Read the model definition and answer for the solid it produces. Units are mm, in the model's axes. A direction names the side the tool comes from. Coordinates: 2 decimals unless noted, no trailing zeros. Write each loop counter-clockwise with the first axis right and the second up, starting at its lowest first coordinate (ties: lowest second). Pieces come first, ordered by that corner, then holes. Notation, with made-up numbers: M 70.25,3.25 L 109.25,3.25 A20 ccw 109.25,26.25 Z; hole C -21,69 d4. An arc over 180 degrees is marked long. Write item = value, one per line.
from build123d import *

# Parameters (mm, degrees)
SKETCH1_W           = 61
SKETCH1_H           = 57
BOSS_EXTRUDE1_DEPTH = 2
FILLET1_R           = 2.5
SKETCH2_R           = 1.25
CUT_EXTRUDE1_DEPTH  = 2
SKETCH3_W           = 31
SKETCH3_H           = 1
CUT_EXTRUDE2_DEPTH  = 2


with BuildPart() as part:
    # Sketch1 → Boss-Extrude1 (new body)
    with BuildSketch(Plane.XY):
        Rectangle(SKETCH1_W, SKETCH1_H)
    extrude(amount=BOSS_EXTRUDE1_DEPTH)

    # Fillet1
    fillet1_edges = [part.edges().sort_by_distance(p)[0] for p in [
        (30.5, -28.5, 1),
        (-30.5, -28.5, 1),
        (-30.5, 28.5, 1),
        (30.5, 28.5, 1),
    ]]
    fillet(fillet1_edges, radius=FILLET1_R)

    # Sketch2 → Cut-Extrude1 (cut)
    with BuildSketch(Plane.XY.offset(2)):
        with Locations((-26.25, 24.5)):
            Circle(SKETCH2_R)
        with Locations((-8.75, 24.5)):
            Circle(SKETCH2_R)
        with Locations((8.75, 24.5)):
            Circle(SKETCH2_R)
        with Locations((26.25, 24.5)):
            Circle(SKETCH2_R)
        with Locations((26.25, 8.166666667)):
            Circle(SKETCH2_R)
        with Locations((26.25, -8.166666667)):
            Circle(SKETCH2_R)
        with Locations((-8.75, -24.5)):
            Circle(SKETCH2_R)
        with Locations((8.75, -24.5)):
            Circle(SKETCH2_R)
        with Locations((26.25, -24.5)):
            Circle(SKETCH2_R)
        with Locations((-26.25, 8.166666667)):
            Circle(SKETCH2_R)
        with Locations((-26.25, -8.166666667)):
            Circle(SKETCH2_R)
        with Locations((-26.25, -24.5)):
            Circle(SKETCH2_R)
    extrude(amount=-CUT_EXTRUDE1_DEPTH, mode=Mode.SUBTRACT)

    # Sketch3 → Cut-Extrude2 (cut)
    with BuildSketch(Plane.XY.offset(2)):
        Rectangle(SKETCH3_W, SKETCH3_H)
        with Locations((0, -2.5)):
            Rectangle(SKETCH3_W, SKETCH3_H)
        with Locations((0, -5)):
            Rectangle(SKETCH3_W, SKETCH3_H)
        with Locations((0, -7.5)):
            Rectangle(SKETCH3_W, SKETCH3_H)
        with Locations((0, -10)):
            Rectangle(SKETCH3_W, SKETCH3_H)
    extrude(amount=-CUT_EXTRUDE2_DEPTH, mode=Mode.SUBTRACT)


solid = part.part
Item 1: Find section C-C (x = 26.25). Determine the outline of the cut face in (y, z).
Worked answers:
outline = M -28.5,0 L -25.75,0 L -25.75,2 L -28.5,2 Z; M -23.25,0 L -9.42,0 L -9.42,2 L -23.25,2 Z; M -6.92,0 L 6.92,0 L 6.92,2 L -6.92,2 Z; M 9.42,0 L 23.25,0 L 23.25,2 L 9.42,2 Z; M 25.75,0 L 28.5,0 L 28.5,2 L 25.75,2 Z
Item 2: Find section A-A (x = -8.75). State how many separate pieces and enclosed holes the cut face has, and give its area (3 significant figures).
Worked answers:
separate_pieces = 8
enclosed_holes = 0
area = 94.0 mm²
Item 3: For a pull along Y with two mould halves and no side action, classify faces 3 (the face through (30.5, 0, 1)), 4 (the face through (7.76, -25.26, 1.01)), 5 (the face through (-29.787, 27.748, 1.014)) as released by +Y, released by -Y, zero draft, split by the parting line, or undercut.
Worked answers:
face_3 = zero draft
face_4 = undercut
face_5 = released by +Y
Item 4: Consider line 1 along Y through (x, z) = (11, 0.85); line 2 along Y through (x, z) = (26.25, 0.7); line 3 along X through (y, z) = (-25.5, 1.8). Determine where each line is inside the solid, lowest interval first. Write a range as from..to.
Worked answers:
line_1 = -28.5..-10.5, -9.5..-8, -7..-5.5, -4.5..-3, -2..-0.5, 0.5..28.5
line_2 = -28.5..-25.75, -23.25..-9.42, -6.92..6.92, 9.42..23.25, 25.75..28.5
line_3 = -30.5..-27, -25.5..-9.5, -8..8, 9.5..25.5, 27..30.5
Item 5: Which of the six approach directions +Z, -Z, +X, -X, +Y, -Y give full straight-line access (tool end or side, diameter ignored) to faces 1 (the face through (0, 0.5, 1)), 2 (the face through (-30.5, 0, 1))?
Worked answers:
face_1 = +Z, -Z
face_2 = +Z, -Z, -X, +Y, -Y
Item 6: A flat-ended cylindrical pin translates along its axis: pin 1 (2 mm diameter, centred on x = 8.75, y = -24.5, fed in from -Z). Find the tip coordinate at first contact, or state that the pin passes through.
Worked answers:
pin_1 = through
Item 7: Find section B-B (y = 24.5). Determine the outline of the cut face in (x, z), and give its area (3 significant figures).
Worked answers:
outline = M -30.5,0 L -27.5,0 L -27.5,2 L -30.5,2 Z; M -25,0 L -10,0 L -10,2 L -25,2 Z; M -7.5,0 L 7.5,0 L 7.5,2 L -7.5,2 Z; M 10,0 L 25,0 L 25,2 L 10,2 Z; M 27.5,0 L 30.5,0 L 30.5,2 L 27.5,2 Z
area = 102 mm²
